The drawing under review shows one solid part. Ordinate dimensions are in mm from its lowest x, y, z. Coordinates: 2 decimals unless noted, no trailing zeros. Loops run counter-clockwise (first coordinate to the right, second up) from the corner with the lowest first, then second, coordinate; pieces in that order, holes last. Notation, with made-up numbers: (34, 1) - (51, 1) arc R20 cw to (51, 20) - close; hole circle Ø9 at (14, -17). An arc over 180 degrees is marked (long way). Answer as a JSON object with one key per item and string values. Group by question number.
Item 1: We need section B-B (z = 4). State how many separate pieces and enclosed holes the cut face has, then the cut area to 3 significant figures.
Item 2: We need section A-A (y = 23.5). Give the boundary of the cut face in (x, z).
Item 3: To check wall thickness, follow line 1 (Y direction, x = 90, z = 0.5); line 2 (X direction, y = 95.5, z = 1); line 3 (Y direction, x = 88, z = 5.5) (1 decimal). State the ranges of each line that lie inside material, in increasing order.
Item 4: We need section C-C (y = 103). Give the boundary of the cut face in (x, z), then the cut area to 3 significant figures.
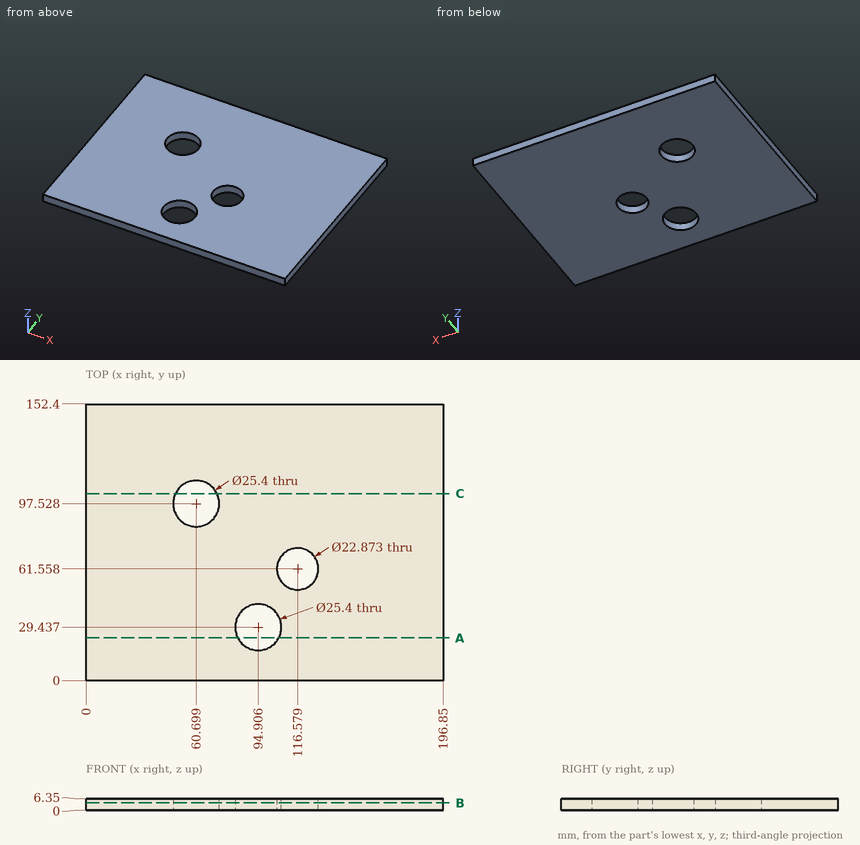
Check sheet entries:
{
 "1": {"separate pieces": "1", "enclosed holes": "3", "area": "28,600 mm2"},
 "2": {"outline": "(0, 0) - (83.68, 0) - (83.68, 6.35) - (0, 6.35) - close; (106.13, 0) - (196.85, 0) - (196.85, 6.35) - (106.13, 6.35) - close"},
 "3": {"line 1": "y = 0 to 17.72, 41.15 to 152.4", "line 2": "x = 0 to 48.16, 73.24 to 196.85", "line 3": "y = 0 to 18.8, 40.1 to 152.4"},
 "4": {"outline": "(0, 0) - (49.24, 0) - (49.24, 6.35) - (0, 6.35) - close; (72.16, 0) - (196.85, 0) - (196.85, 6.35) - (72.16, 6.35) - close", "area": "1,100 mm2"}
}
